The model under review builds one solid part; all positions refer to its coordinate system, in mm. Face numbers are marked on the shaded views. A direction names the side the tool comes from. Coordinates: 2 decimals unless noted, no trailing zeros. Order: outer loops, then holes, each group sorted by start corner. A loop starts at its lowest first (then second) coordinate and runs counter-clockwise, first axis right, second up. Notation, with made-up numbers: (-40, 35.5) -> (-27, 35.5) arc R36 cw to (-27, 70.5) -> close; hole circle Ø11 at (-36, 66.5). An arc over 180 degrees is marked (long way). Use one line per item in the form item = value.
from build123d import *

# Parameters (mm, degrees)
F2_SIZE   = 0.3
F3_SIZE   = 0.3
F4_SIZE   = 0.3
F7_W      = 6
F7_H      = 6
F8_DEPTH  = 1.1
F10_W     = 6
F10_H     = 6
F11_DEPTH = 1.1
F13_D     = 5
F13_DEPTH = 15
F13_TIP   = 1.5021515476


with BuildPart() as f1:
    # F0 (on Front) → F1 (revolve)
    with BuildSketch(Plane.XZ):
        Polygon((-26.3235288649, 4.5), (-26.3235288649, 0), (33.6764711351, 0), (33.6764711351, 4.5), (-2.3235288649, 4.5), (-2.3235288649, 8), (-16.3235288649, 8), (-16.3235288649, 4.5), align=None)
    revolve(axis=Axis((3.6764711351, 0, 0), (1, 0, 0)))

    # F2
    f2_edges = [f1.edges().sort_by_distance(p)[0] for p in [
        (33.676471, 0, -4.5),
    ]]
    chamfer(f2_edges, length=F2_SIZE)

    # F3
    f3_edges = [f1.edges().sort_by_distance(p)[0] for p in [
        (-2.323529, 0, -8),
        (-16.323529, 0, -8),
        (-9.323529, 0, 8),
    ]]
    chamfer(f3_edges, length=F3_SIZE)

    # F4
    f4_edges = [f1.edges().sort_by_distance(p)[0] for p in [
        (-26.323529, 0, -4.5),
    ]]
    chamfer(f4_edges, length=F4_SIZE)

    # F7 (on offset) → F8 (cut)
    with BuildSketch(Plane.XZ.offset(4.5)):
        with Locations((12.6764711351, 0)):
            Rectangle(F7_W, F7_H)
    extrude(amount=-F8_DEPTH, mode=Mode.SUBTRACT)

    # F10 (on offset) → F11 (cut)
    with BuildSketch(Plane.XY.offset(4.5)):
        with Locations((12.6764711351, 0)):
            Rectangle(F10_W, F10_H)
    extrude(amount=-F11_DEPTH, mode=Mode.SUBTRACT)

    # F13
    with Locations(Plane(origin=(-26.3235288649, 0, 0), x_dir=(0, -1, 0), z_dir=(-1, 0, 0))):
        with Locations((0, 0)):
            Hole(F13_D / 2, depth=F13_DEPTH)
            with Locations((0, 0, -(F13_DEPTH + F13_TIP / 2))):  # 118° drill point
                Cone(0, F13_D / 2, F13_TIP, mode=Mode.SUBTRACT)


solid = f1.part
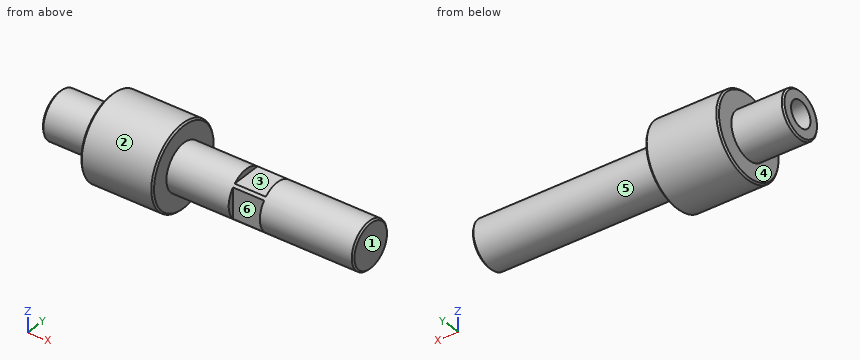
Item 1: Draft analysis for pull direction X (two halves, no side actions). For the marked faces 1, 2 and 3, state which applies: released by +X, released by -X, zero draft, split by the parting line, or undercut.
Results found:
face_1 = released by +X
face_2 = zero draft
face_3 = undercut
Item 2: Clearance check with flat-ended pins moving along their axes: pin 1 (8 mm diameter, centred on x = -10.5, y = -5, fed in from +Z); pin 2 (2 mm diameter, centred on x = -3, y = 5, fed in from +Z); pin 3 (4.5 mm diameter, centred on x = 11.5, z = -1.5, fed in from -Y); pin 4 (7.5 mm diameter, centred on y = -3.5, z = 3.5, fed in from +X). State where each tip first meets the part, or that it passes through.
Results found:
pin_1 = 7.94
pin_2 = 6.93
pin_3 = -4.5
pin_4 = 33.68
Item 3: We need section B-B (x = -4.5). Write out the cut boundary in (y, z), plus the area to 3 significant figures.
Results found:
outline = circle Ø16 at (0, 0)
area = 201 mm²
Item 4: To check wall thickness, follow L1, parallel to Z at x = -21.25, y = 0; L2, parallel to Y at x = -14.75, z = 0; L3, parallel to X at y = -7, z = -0.25. State the ranges of each line that lie inside material, in increasing order. Write a range as from..to.
Results found:
L1 = -4.5..-2.5, 2.5..4.5
L2 = -8..-2.5, 2.5..8
L3 = -16.32..-2.32
Item 5: Tool access review of the marked faces 4, 5 and 6: name each direction out of +Z, -Z, +X, -X, +Y, -Y from which nothing blocks a thin tool from reaching the whole face with its end or side.
Results found:
face_4 = -X
face_5 = +X
face_6 = +Z, -Z, -Y
Item 6: We need section C-C (x = 8). Write out the cut boundary in (y, z).
Results found:
outline = circle Ø9 at (0, 0)
Item 7: We need section A-A (x = -12). Write out the cut boundary in (y, z).
Results found:
outline = circle Ø16 at (0, 0); hole circle Ø5 at (0, 0)
